Build history of the part. All positions in model axes, mm. Face numbers are marked on the shaded views. A direction names the side the tool comes from. Round coordinates to 2 decimals unless told otherwise and drop trailing zeros. Write each loop counter-clockwise with the first axis right and the second up, starting at its lowest first coordinate (ties: lowest second). Pieces come first, ordered by that corner, then holes.
1) Which spindle directions (+Z, -Z, +X, -X, +Y, -Y) get a long thin tool onto all of the face, cutting with end or side? Do the marked faces 4, 5 and 6. Say none if no direction does.
2) Saw through at A-A (x = 1). Write the cut outline in (y, z) (3 decimals).
3) Pull direction Z, two halves, no side cores. Call the marked faces 1, 2 and 3: +Z half, -Z half, draft (parallel to the pull), parting line (faces both ways), or undercut.
4) Wall check: probe 1 along Y at (x, z) = (0.9, 0) (3 decimals); probe 2 along Y at (x, z) = (1.8, 0) (3 decimals); probe 3 along X at (y, z) = (-1.75, 3.75). Give the ranges that are in metal, low to high.
5) Flat gauge pins, fed straight in: pin 1 (4 mm diameter, centred on x = -9, z = -1.5, fed in from +Y); pin 2 (3.5 mm diameter, centred on y = 0, z = 0, fed in from +X); pin 3 (4 mm diameter, centred on x = 16.5, y = 3, fed in from -Z); pin 4 (1.5 mm diameter, centred on x = 7, y = -0.5, fed in from +Z). Where does each tip first touch, or does it go through?
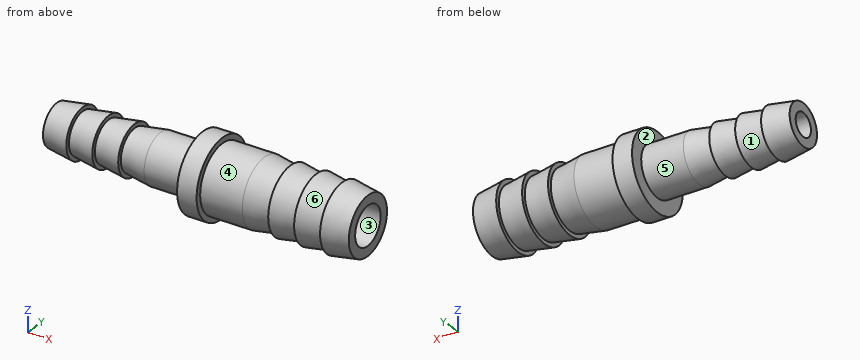
from build123d import *

# Parameters (mm, degrees)
SKETCH1_W       = 25.273
SKETCH1_H       = 2.159
SKETCH2_W       = 3.175
SKETCH2_H       = 4.445
LPATTERN1_COUNT = 4
LPATTERN1_PITCH = 4.212166667
SKETCH4_W       = 25.273
SKETCH4_H       = 2.286
LPATTERN2_COUNT = 4
LPATTERN2_PITCH = 4.212166667
SKETCH6_W       = 2.032
SKETCH6_H       = 1.27


with BuildPart() as part:
    # Sketch1 → Revolve1 (revolve)
    with BuildSketch(Plane.XY, mode=Mode.PRIVATE) as revolve1_sk:
        with Locations((-12.6365, 2.9845)):
            Rectangle(SKETCH1_W, SKETCH1_H)
    revolve(revolve1_sk.sketch.rotate(Axis((-25.273, 0, 0), (1, 0, 0)), 90), axis=Axis((-25.273, 0, 0), (1, 0, 0)))

    # Sketch2 → Revolve2 (revolve)
    with BuildSketch(Plane.XY, mode=Mode.PRIVATE) as revolve2_sk:
        with Locations((0, 4.1275)):
            Rectangle(SKETCH2_W, SKETCH2_H)
    revolve(revolve2_sk.sketch.rotate(Axis((0, 0, 0), (-1, 0, 0)), 270), axis=Axis((0, 0, 0), (-1, 0, 0)))

    # Sketch3 → Cut-Revolve1 (revolve, cut)
    with BuildSketch(Plane.XY, mode=Mode.PRIVATE) as cut_revolve1_sk:
        Polygon((-25.273, 4.064), (-25.273, 3.4163), (-21.060833333, 4.064), align=None)
    cut_revolve1 = revolve(cut_revolve1_sk.sketch.rotate(Axis((-25.273, 0, 0), (1, 0, 0)), 90), axis=Axis((-25.273, 0, 0), (1, 0, 0)), mode=Mode.SUBTRACT)

    # LPattern1: Cut-Revolve1 ×4
    with Locations(*[(i * LPATTERN1_PITCH, 0, 0) for i in range(1, LPATTERN1_COUNT)]):
        add(cut_revolve1, mode=Mode.SUBTRACT)



with BuildPart() as body_2:
    # Sketch4 → Revolve3 (revolve)
    with BuildSketch(Plane.XY, mode=Mode.PRIVATE) as revolve3_sk:
        with Locations((12.6365, 4.318)):
            Rectangle(SKETCH4_W, SKETCH4_H)
    revolve(revolve3_sk.sketch.rotate(Axis((0, 0, 0), (1, 0, 0)), 90), axis=Axis((0, 0, 0), (1, 0, 0)))

    # Sketch5 → Cut-Revolve2 (revolve, cut)
    with BuildSketch(Plane.XY, mode=Mode.PRIVATE) as cut_revolve2_sk:
        Polygon((25.273, 5.461), (25.273, 4.7752), (21.060833333, 5.461), align=None)
    cut_revolve2 = revolve(cut_revolve2_sk.sketch.rotate(Axis((-25.273, 0, 0), (1, 0, 0)), 90), axis=Axis((-25.273, 0, 0), (1, 0, 0)), mode=Mode.SUBTRACT)

    # LPattern2: Cut-Revolve2 ×4
    with Locations(*[(-i * LPATTERN2_PITCH, 0, 0) for i in range(1, LPATTERN2_COUNT)]):
        add(cut_revolve2, mode=Mode.SUBTRACT)


with BuildPart() as part_1:
    add(part.part)

    add(body_2.part)  # Revolve4 merges body 2
    # Sketch6 → Revolve4 (revolve)
    with BuildSketch(Plane.XY, mode=Mode.PRIVATE) as revolve4_sk:
        with Locations((1.016, 2.54)):
            Rectangle(SKETCH6_W, SKETCH6_H)
    revolve(revolve4_sk.sketch.rotate(Axis((-25.273, 0, 0), (1, 0, 0)), 90), axis=Axis((-25.273, 0, 0), (1, 0, 0)))


solid = part_1.part
Evaluation:
1. face 4: +X
1. face 5: -X
1. face 6: none
2. outline: circle Ø12.7 at (0, 0); hole circle Ø3.81 at (0, 0)
3. face 1: parting line
3. face 2: draft
3. face 3: undercut
4. probe 1: y = -6.35 to -1.905, 1.905 to 6.35
4. probe 2: y = -5.461 to -1.905, 1.905 to 5.461
4. probe 3: x = -1.59 to 25.27
5. pin 1: stops at y = 4.06
5. pin 2: passes through
5. pin 3: stops at z = -5.36
5. pin 4: stops at z = 5.46
